For this review, take the finished solid that the model builds, in its own axes (mm). A direction names the side the tool comes from. Round coordinates to 2 decimals unless told otherwise and drop trailing zeros. Order: outer loops, then holes, each group sorted by start corner. A loop starts at its lowest first (then second) coordinate and runs counter-clockwise, first axis right, second up.
from build123d import *

# Parameters (mm, degrees)
F0_W     = 5.08
F0_H     = 0.762
F0_W_2   = 2.413
F2_W     = 76.2
F2_H     = 76.2
F3_DEPTH = 0.762
F4_R     = 5.08


with BuildPart() as f1:
    # F0 (on Right) → F1 (revolve)
    with BuildSketch(Plane.YZ):
        with Locations((-27.94, 3.683)):
            Rectangle(F0_W, F0_H)
        Polygon((-25.4, 3.302), (-19.05, 0), (-19.05, 0.762), (-25.4, 4.064), align=None)
        with Locations((-17.8435, 0.381)):
            Rectangle(F0_W_2, F0_H)
    revolve(axis=Axis((0, 0, 0.2757511821), (0, 0, 1)))

    # F2 (on face) → F3 (join, through all)
    with BuildSketch(Plane.XY.offset(4.064)):
        Rectangle(F2_W, F2_H)
        with BuildLine():
            ThreePointArc((-32.512, 30.48), (-34.3893232101, 31.7343872654), (-33.9488409794, 33.9488409794))
            ThreePointArc((-33.9488409794, 33.9488409794), (-31.7343872654, 34.3893232101), (-30.48, 32.512))
            Line((-30.48, 32.512), (30.48, 32.512))
            ThreePointArc((30.48, 32.512), (32.512, 34.544), (34.544, 32.512))
            ThreePointArc((34.544, 32.512), (33.9488409794, 31.0751590206), (32.512, 30.48))
            Line((32.512, 30.48), (32.512, -30.48))
            ThreePointArc((32.512, -30.48), (33.9488409794, -31.0751590206), (34.544, -32.512))
            ThreePointArc((34.544, -32.512), (32.512, -34.544), (30.48, -32.512))
            Line((30.48, -32.512), (-30.48, -32.512))
            ThreePointArc((-30.48, -32.512), (-33.9488409794, -33.9488409794), (-32.512, -30.48))
            Line((-32.512, -30.48), (-32.512, 30.48))
        make_face(mode=Mode.SUBTRACT)
        with BuildLine():
            Line((30.48, 32.512), (-30.48, 32.512))
            ThreePointArc((-30.48, 32.512), (-30.6346767899, 31.7343872654), (-31.0751590206, 31.0751590206))
            ThreePointArc((-31.0751590206, 31.0751590206), (-31.7343872654, 30.6346767899), (-32.512, 30.48))
            Line((-32.512, 30.48), (-32.512, -30.48))
            ThreePointArc((-32.512, -30.48), (-31.0751590206, -31.0751590206), (-30.48, -32.512))
            Line((-30.48, -32.512), (30.48, -32.512))
            ThreePointArc((30.48, -32.512), (31.0751590206, -31.0751590206), (32.512, -30.48))
            Line((32.512, -30.48), (32.512, 30.48))
            ThreePointArc((32.512, 30.48), (31.0751590206, 31.0751590206), (30.48, 32.512))
        make_face()
        with BuildLine():
            ThreePointArc((-27.051, 25.8572), (-28.1539273859, 26.5941525184), (-27.8951440754, 27.8951440754))
            ThreePointArc((-27.8951440754, 27.8951440754), (-26.5941525184, 28.1539273859), (-25.8572, 27.051))
            Line((-25.8572, 27.051), (-14.0454191465, 27.051))
            ThreePointArc((-14.0454191465, 27.051), (0, 30.48), (14.0454191465, 27.051))
            Line((14.0454191465, 27.051), (25.8572, 27.051))
            ThreePointArc((25.8572, 27.051), (27.051, 28.2448), (28.2448, 27.051))
            ThreePointArc((28.2448, 27.051), (27.8951440754, 26.2068559246), (27.051, 25.8572))
            Line((27.051, 25.8572), (27.051, 14.0454191465))
            ThreePointArc((27.051, 14.0454191465), (29.6103434631, 7.2289667311), (30.48, 0))
            ThreePointArc((30.48, 0), (29.6103434631, -7.2289667311), (27.051, -14.0454191465))
            Line((27.051, -14.0454191465), (27.051, -25.8572))
            ThreePointArc((27.051, -25.8572), (27.8951440754, -26.2068559246), (28.2448, -27.051))
            ThreePointArc((28.2448, -27.051), (27.051, -28.2448), (25.8572, -27.051))
            Line((25.8572, -27.051), (14.0454191465, -27.051))
            ThreePointArc((14.0454191465, -27.051), (0, -30.48), (-14.0454191465, -27.051))
            Line((-14.0454191465, -27.051), (-25.8572, -27.051))
            ThreePointArc((-25.8572, -27.051), (-27.8951440754, -27.8951440754), (-27.051, -25.8572))
            Line((-27.051, -25.8572), (-27.051, -14.0454191465))
            ThreePointArc((-27.051, -14.0454191465), (-30.48, 0), (-27.051, 14.0454191465))
            Line((-27.051, 14.0454191465), (-27.051, 25.8572))
        make_face(mode=Mode.SUBTRACT)
        with BuildLine():
            Line((27.051, -25.8572), (27.051, -14.0454191465))
            ThreePointArc((27.051, -14.0454191465), (21.5526146906, -21.5526146906), (14.0454191465, -27.051))
            Line((14.0454191465, -27.051), (25.8572, -27.051))
            ThreePointArc((25.8572, -27.051), (26.2068559246, -26.2068559246), (27.051, -25.8572))
        make_face()
        with BuildLine():
            Line((25.8572, 27.051), (14.0454191465, 27.051))
            ThreePointArc((14.0454191465, 27.051), (21.5526146906, 21.5526146906), (27.051, 14.0454191465))
            Line((27.051, 14.0454191465), (27.051, 25.8572))
            ThreePointArc((27.051, 25.8572), (26.2068559246, 26.2068559246), (25.8572, 27.051))
        make_face()
        with BuildLine():
            ThreePointArc((-14.0454191465, -27.051), (-21.5526146906, -21.5526146906), (-27.051, -14.0454191465))
            Line((-27.051, -14.0454191465), (-27.051, -25.8572))
            ThreePointArc((-27.051, -25.8572), (-26.2068559246, -26.2068559246), (-25.8572, -27.051))
            Line((-25.8572, -27.051), (-14.0454191465, -27.051))
        make_face()
        with BuildLine():
            ThreePointArc((-26.2068559246, 26.2068559246), (-26.5941525184, 25.9480726141), (-27.051, 25.8572))
            Line((-27.051, 25.8572), (-27.051, 14.0454191465))
            ThreePointArc((-27.051, 14.0454191465), (-24.589984475, 18.0100822741), (-21.5526146906, 21.5526146906))
            Line((-21.5526146906, 21.5526146906), (-26.2068559246, 26.2068559246))
        make_face()
        with BuildLine():
            Line((-14.0454191465, 27.051), (-25.8572, 27.051))
            ThreePointArc((-25.8572, 27.051), (-25.9480726141, 26.5941525184), (-26.2068559246, 26.2068559246))
            Line((-26.2068559246, 26.2068559246), (-21.5526146906, 21.5526146906))
            ThreePointArc((-21.5526146906, 21.5526146906), (-18.0100822741, 24.589984475), (-14.0454191465, 27.051))
        make_face()
    extrude(amount=-F3_DEPTH)

    # F4
    f4_edges = [f1.edges().sort_by_distance(p)[0] for p in [
        (-38.1, -38.1, 3.683),
        (38.1, -38.1, 3.683),
        (-38.1, 38.1, 3.683),
        (38.1, 38.1, 3.683),
    ]]
    fillet(f4_edges, radius=F4_R)


solid = f1.part
(1) Add section A-A on x = 0. Give the boundary of the cut face in (y, z), plus the area to 3 significant figures.
(2) Clearance check with flat-ended pins moving along their axes: P1, Ø1, axis at x = -4, z = 1, coming from the +Y side; P2, Ø5.5, axis at x = -32.512, y = -32.512, coming from the +Z side; P3, Ø1, axis at x = 26.5, z = 1, coming from the -Y side; P4, Ø1, axis at x = 7.5, z = 2.5, coming from the +Y side. State where each tip first meets the part, or that it passes through.
(3) Wall thickness on L1, parallel to Z at x = 34, y = 11; L2, parallel to X at y = -12, z = 3.85; L3, parallel to Y at x = 8.5, z = 1.25: over which ranges is each line inside the solid? List them lowest first.
(4) Draft analysis for pull direction X (two halves, no side actions). For faces 1 (the face through (-36.651, 36.572, 3.678)), 2 (the face through (-1, 26, 4.064)), 3 (the face through (36.572, -36.651, 3.678)), 4 (the face through (-18.985, 4.216, 0.969)), state which applies: pulls with the +X half, pulls with the -X half, needs draft (parallel to the pull), parting line crosses it, or undercut.
(5) Add section C-C on z = 1.4. Give the boundary of the cut face in (x, y).
(6) Tool access review of faces 5 (the face through (-17, 0, 0.762)), 6 (the face through (-1, 26, 3.302)), 7 (the face through (36.572, 36.651, 3.678)): name each direction out of +Z, -Z, +X, -X, +Y, -Y from which nothing blocks a thin tool from reaching the whole face with its end or side.
Here are the results:
1. outline: (-38.1, 3.3) - (-25.4, 3.3) - (-19.05, 0) - (-16.64, 0) - (-16.64, 0.76) - (-19.05, 0.76) - (-25.4, 4.06) - (-38.1, 4.06) - close; (16.64, 0) - (19.05, 0) - (25.4, 3.3) - (38.1, 3.3) - (38.1, 4.06) - (25.4, 4.06) - (19.05, 0.76) - (16.64, 0.76) - close
1. area: 32.7 mm2
2. P1: stops at y = 21.57
2. P2: stops at z = 4.06
2. P3: passes through
2. P4: stops at y = 23.67
3. L1: z = 3.3 to 4.06
3. L2: x = -38.1 to -21.92, 21.92 to 38.1
3. L3: y = -19.7 to -18.09, 18.09 to 19.7
4. face 1: pulls with the -X half
4. face 2: needs draft
4. face 3: pulls with the +X half
4. face 4: undercut
5. outline: circle Ø43.48 at (0, 0); hole circle Ø40.55 at (0, 0)
6. face 5: +Z
6. face 6: -Z
6. face 7: +Z, -Z, +X, +Y
